Can you work these out from the drawing? Everything is in mm from the part's minimum corner. Coordinates: 2 decimals unless noted, no trailing zeros. Order: outer loops, then holes, each group sorted by start corner. A loop starts at its lowest first (then second) coordinate and runs counter-clockwise, first axis right, second up. Notation, with made-up numbers: (81.5, 29) -> (129.5, 29) arc R18 ccw to (129.5, 48) -> close; hole circle Ø2 at (80.5, -6.75). An arc over 180 degrees is marked (long way). Return JSON: item names as keys, results as strings. Group by question number.
1) For pin 1 (1.5 mm diameter, centred on x = 6, y = 55, fed in from +Z); pin 2 (5 mm diameter, centred on x = 6, y = 35.5, fed in from +Z); pin 3 (5 mm diameter, centred on x = 7.5, y = 6.5, fed in from +Z), each with a flat end and sliding along its axis, tell me the tip position at first contact or that it passes through.
2) If I drill on probe 1 along Z at (x, y) = (10.5, 14); probe 2 along Z at (x, y) = (13.5, 11.5), over which ranges is the centre line in solid material (lowest first)? Write a range as from..to.
3) If we section it at A-A, the plane x = 3.75: Please give me the cut outline in (y, z).
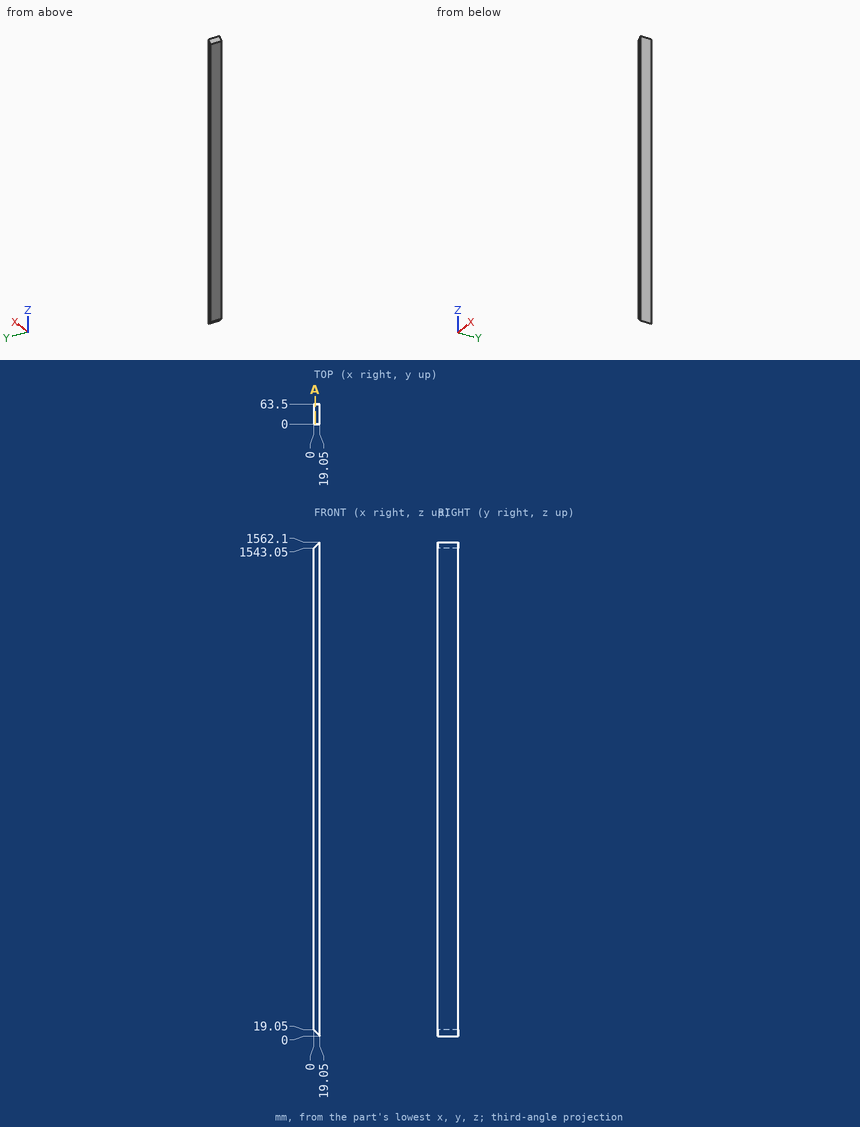
Result sheet:
{
 "1": {"pin 1": "stops at z = 1549.8", "pin 2": "stops at z = 1551.55", "pin 3": "stops at z = 1553.05"},
 "2": {"probe 1": "z = 8.55..1553.55", "probe 2": "z = 5.55..1556.55"},
 "3": {"outline": "(0, 15.3) -> (63.5, 15.3) -> (63.5, 1546.8) -> (0, 1546.8) -> close"}
}
